Geometry check sheet. Reference: the model listing, model coordinates, mm. A direction names the side the tool comes from. Round coordinates to 2 decimals unless told otherwise and drop trailing zeros. Return JSON: item names as keys, results as strings.
```python
from build123d import *

# Parameters (mm, degrees)
ESQUISSE1_W                        = 30
ESQUISSE1_H                        = 30
BOSS_EXTRU_1_DEPTH                 = 2
BOSS_EXTRU_5_DEPTH                 = 10
CONG_1_R                           = 1
ESQUISSE2_R                        = 3.6
BOSS_EXTRU_6_DEPTH                 = 5
R_P_TITION_CIRCULAIRE1_COUNT       = 4
CONG_1_OF_R_P_TITION_CIRCULAIRE1_R = 1
CONG_2_R                           = 2
CONG_3_R                           = 1
CONG_4_R                           = 2


with BuildPart() as part:
    # Esquisse1 → Boss.-Extru.1 (new body)
    with BuildSketch(Plane.XY):
        with Locations((15, 15)):
            Rectangle(ESQUISSE1_W, ESQUISSE1_H)
    extrude(amount=BOSS_EXTRU_1_DEPTH)

    # Esquisse5 → Boss.-Extru.5 (add)
    with BuildSketch(Plane.XY.offset(2)):
        Polygon((27.7, 6.4), (27.7, 23.6), (25.05, 23.6), (21.6, 19.2), (21.6, 10.8), (25.05, 6.4), align=None)
    boss_extru_5 = extrude(amount=BOSS_EXTRU_5_DEPTH)

    # Congé1
    cong_1_edges = [part.edges().sort_by_distance(p)[0] for p in [
        (25.05, 6.4, 7),
        (27.7, 6.4, 7),
        (27.7, 23.6, 7),
        (25.05, 23.6, 7),
        (21.6, 19.2, 7),
        (21.6, 10.8, 7),
    ]]
    fillet(cong_1_edges, radius=CONG_1_R)

    # Esquisse2 → Boss.-Extru.6 (add)
    with BuildSketch(Plane.XY.offset(2)):
        with Locations(Location((15, 15, 0), (0, 0, 180))):
            Circle(ESQUISSE2_R)
    extrude(amount=BOSS_EXTRU_6_DEPTH)

    # Répétition circulaire1: Boss.-Extru.5 ×4 about axis
    r_p_tition_circulaire1_axis = Axis((15, 15, 0), (0, 0, 1))
    for i in range(1, R_P_TITION_CIRCULAIRE1_COUNT):
        add(boss_extru_5.rotate(r_p_tition_circulaire1_axis, i * 360 / R_P_TITION_CIRCULAIRE1_COUNT))

    # Congé1 of Répétition circulaire1
    cong_1_of_r_p_tition_circulaire1_edges = [part.edges().sort_by_distance(p)[0] for p in [
        (23.6, 25.05, 7),
        (23.6, 27.7, 7),
        (6.4, 27.7, 7),
        (6.4, 25.05, 7),
        (10.8, 21.6, 7),
        (19.2, 21.6, 7),
        (4.95, 23.6, 7),
        (2.3, 23.6, 7),
        (2.3, 6.4, 7),
        (4.95, 6.4, 7),
        (8.4, 10.8, 7),
        (8.4, 19.2, 7),
        (6.4, 4.95, 7),
        (6.4, 2.3, 7),
        (23.6, 2.3, 7),
        (23.6, 4.95, 7),
        (19.2, 8.4, 7),
        (10.8, 8.4, 7),
    ]]
    fillet(cong_1_of_r_p_tition_circulaire1_edges, radius=CONG_1_OF_R_P_TITION_CIRCULAIRE1_R)

    # Congé2
    cong_2_edges = [part.edges().sort_by_distance(p)[0] for p in [
        (0, 30, 1),
        (30, 30, 1),
        (30, 0, 1),
        (0, 0, 1),
    ]]
    fillet(cong_2_edges, radius=CONG_2_R)

    # Congé3
    cong_3_edges = [part.edges().sort_by_distance(p)[0] for p in [
        (15, 27.7, 12),
        (23.6, 26.118328167, 12),
        (6.4, 26.118328167, 12),
        (8.655619048, 23.28138961, 12),
        (15, 21.6, 12),
        (21.344380952, 23.28138961, 12),
        (6.500824998, 25.099067124, 12),
        (10.818910387, 21.654764961, 12),
        (19.181089613, 21.654764961, 12),
        (23.499175002, 25.099067124, 12),
        (6.692893219, 27.407106781, 12),
        (23.307106781, 27.407106781, 12),
        (2.3, 15, 12),
        (3.881671833, 23.6, 12),
        (3.881671833, 6.4, 12),
        (6.71861039, 8.655619048, 12),
        (8.4, 15, 12),
        (6.71861039, 21.344380952, 12),
        (4.900932876, 6.500824998, 12),
        (8.345235039, 10.818910387, 12),
        (8.345235039, 19.181089613, 12),
        (4.900932876, 23.499175002, 12),
        (2.592893219, 6.692893219, 12),
        (2.592893219, 23.307106781, 12),
        (15, 2.3, 12),
        (6.4, 3.881671833, 12),
        (23.6, 3.881671833, 12),
        (21.344380952, 6.71861039, 12),
        (15, 8.4, 12),
        (8.655619048, 6.71861039, 12),
        (23.499175002, 4.900932876, 12),
        (19.181089613, 8.345235039, 12),
        (10.818910387, 8.345235039, 12),
        (6.500824998, 4.900932876, 12),
        (23.307106781, 2.592893219, 12),
        (6.692893219, 2.592893219, 12),
        (27.7, 15, 12),
        (26.118328167, 6.4, 12),
        (26.118328167, 23.6, 12),
        (23.28138961, 21.344380952, 12),
        (21.6, 15, 12),
        (23.28138961, 8.655619048, 12),
        (25.099067124, 23.499175002, 12),
        (21.654764961, 19.181089613, 12),
        (21.654764961, 10.818910387, 12),
        (25.099067124, 6.500824998, 12),
        (27.407106781, 23.307106781, 12),
        (27.407106781, 6.692893219, 12),
        (18.6, 15, 7),
    ]]
    fillet(cong_3_edges, radius=CONG_3_R)

    # Congé4
    cong_4_edges = [part.edges().sort_by_distance(p)[0] for p in [
        (29.414213562, 29.414213562, 0),
        (15, 30, 0),
        (0.585786438, 29.414213562, 0),
        (0, 15, 0),
        (0.585786438, 0.585786438, 0),
        (15, 0, 0),
        (29.414213562, 0.585786438, 0),
        (30, 15, 0),
    ]]
    fillet(cong_4_edges, radius=CONG_4_R - 0.0001)  # a hair under: the kernel refuses the full size


solid = part.part
```
(1) Release check for a two-part mould opening along X. For faces 6 (the face through (23.6, 26, 6)), 7 (the face through (2.585, 23.299, 6.563)), 8 (the face through (8.68, 6.74, 6.44)) record: pulls with the +X half, pulls with the -X half, needs draft (parallel to the pull), parting line crosses it, or undercut.
Response values:
{"face 6": "pulls with the +X half", "face 7": "pulls with the -X half", "face 8": "undercut"}
(2) Material ranges on line 1 along X through (y, z) = (13.5, 2.5); line 2 along Y through (x, z) = (12.5, 6); line 3 along Y through (x, z) = (7.5, 4), recorded low to high. Write a range as [from, to].
Response values:
{"line 1": "x = [2.3, 8.4], [11.73, 18.27], [21.6, 27.7]", "line 2": "y = [2.3, 8.4], [12.41, 17.59], [21.6, 27.7]", "line 3": "y = [2.3, 5.81], [9.65, 20.35], [24.19, 27.7]"}
(3) Access from +Z, -Z, +X, -X, +Y, -Y to the whole of each face (thin tool, end or side, straight path). Record for faces 1 (the face through (6.4, 26, 6)), 2 (the face through (2.585, 14.894, 11.699)), 3 (the face through (21.32, 23.26, 6.44)), 4 (the face through (26.126, 6.685, 11.699)), 5 (the face through (26.11, 23.315, 11.699)).
Response values:
{"face 1": "+Z, -X, +Y", "face 2": "+Z, -X, +Y, -Y", "face 3": "+Z", "face 4": "+Z, +X, -Y", "face 5": "+Z, +X, +Y"}
(4) Gauge pin test, flat ends, axial feed: pin 1 (1.3 mm diameter, centred on y = 4, z = 5.5, fed in from -X); pin 2 (2.5 mm diameter, centred on y = 15.5, z = 8, fed in from -X); pin 3 (1.3 mm diameter, centred on y = 4, z = 4.5, fed in from +X); pin 4 (5 mm diameter, centred on x = 15.5, z = 3.5, fed in from -Y). Record the tip position at first contact, or that the pin passes through.
Response values:
{"pin 1": "stops at x = 6.4", "pin 2": "stops at x = 2.3", "pin 3": "stops at x = 23.6", "pin 4": "stops at y = 0"}
(5) Section check A-A, the plane z = 5. Give the number of separate pieces and of enclosed holes in the cut face, plus the area to 3 significant figures.
Response values:
{"separate pieces": "5", "enclosed holes": "0", "area": "398 mm^2"}
